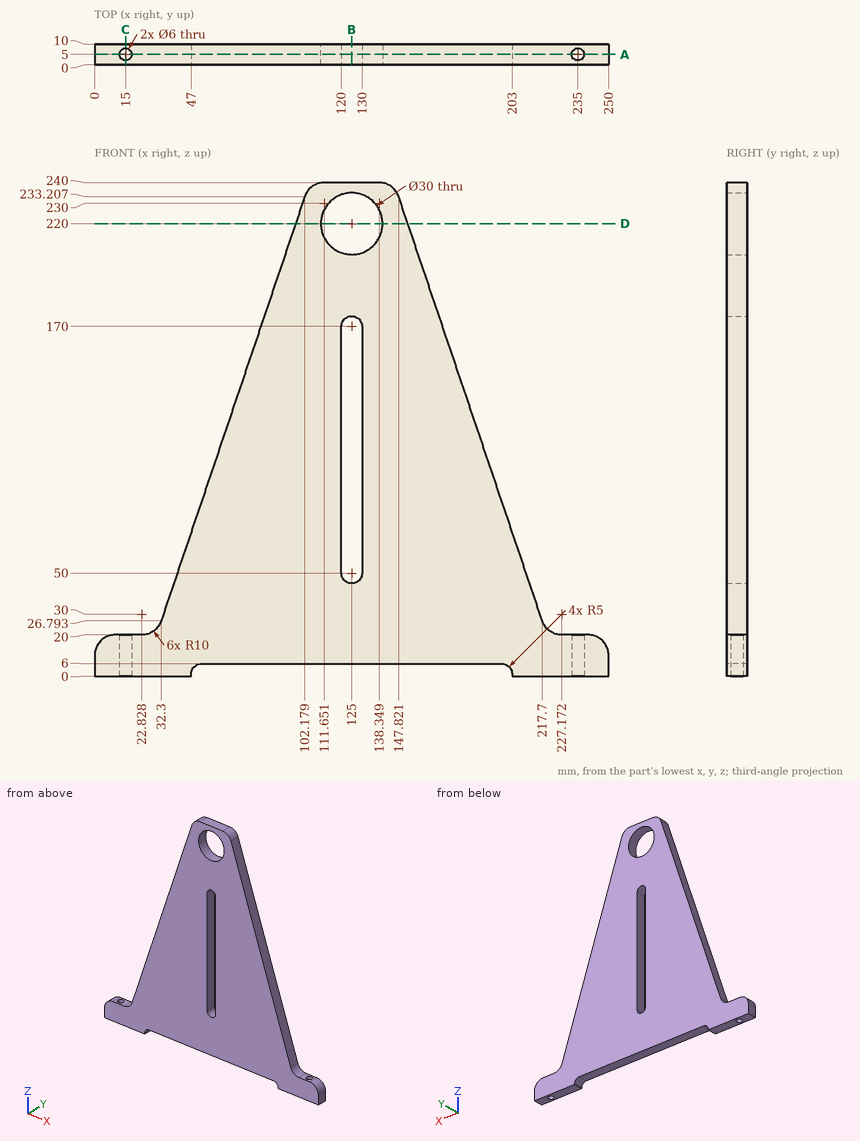
Source: three-view drawing plus pictorial views. Frame: mm from the lowest corner of the part. Coordinates: 2 decimals unless noted, no trailing zeros. Write each loop counter-clockwise with the first axis right and the second up, starting at its lowest first coordinate (ties: lowest second). Pieces come first, ordered by that corner, then holes. Notation, with made-up numbers: (72.5, 48.5) - (82.5, 48.5) arc R20 ccw to (82.5, 68.5) - close; hole circle Ø11 at (50.25, -8.75). An arc over 180 degrees is marked (long way). Return JSON: item names as keys, results as strings.
Item 1: Section query A-A (y = 5). Count the separate pieces of the cut face and the enclosed holes in it, and give its area (3 significant figures).
Completed:
{"separate pieces": "3", "enclosed holes": "2", "area": "27,200 mm2"}
Item 2: Section query C-C (x = 15). Output: boundary loops of the cut face in (y, z).
Completed:
{"outline": "(0, 0) - (2, 0) - (2, 20) - (0, 20) - close; (8, 0) - (10, 0) - (10, 20) - (8, 20) - close"}
Item 3: Pin query (flat end, axial travel): pin 1 Ø1 at (x, y) = (154.5, 3) entering from -Z; pin 2 Ø5 at (x, y) = (236.5, 3) entering from +Z; pin 3 Ø2 at (y, z) = (2.5, 85.5) entering from -X; pin 4 Ø5.5 at (x, y) = (235, 5) entering from -Z. Return the tip coordinate at first contact, or that it passes through.
Completed:
{"pin 1": "stops at z = 6", "pin 2": "stops at z = 20", "pin 3": "stops at x = 51.84", "pin 4": "passes through"}
Item 4: Line query: L1, parallel to Z at x = 125, y = 6.5; L2, parallel to Y at x = 15, z = 6; L3, parallel to Z at x = 20, y = 3.25. Output: solid intervals per line, ascending.
Completed:
{"L1": "z = 6 to 45, 175 to 205, 235 to 240", "L2": "y = 0 to 2, 8 to 10", "L3": "z = 0 to 20"}
Item 5: Section query D-D (z = 220). Output: boundary loops of the cut face in (x, y).
Completed:
{"outline": "(97.71, 0) - (110, 0) - (110, 10) - (97.71, 10) - close; (140, 0) - (152.29, 0) - (152.29, 10) - (140, 10) - close"}
Item 6: Section query B-B (x = 125). Output: boundary loops of the cut face in (y, z).
Completed:
{"outline": "(0, 6) - (10, 6) - (10, 45) - (0, 45) - close; (0, 175) - (10, 175) - (10, 205) - (0, 205) - close; (0, 235) - (10, 235) - (10, 240) - (0, 240) - close"}
